Autodesk Inventor part; units mm, degrees
ref_plane "YZ Plane" through (0, 0, 0) normal (1, 0, 0) x (0, 1, 0)
ref_plane "XZ Plane" through (0, 0, 0) normal (0, 1, 0) x (-1, 0, 0)
ref_plane "XY Plane" through (0, 0, 0) normal (0, 0, 1) x (1, 0, 0)
sketch "Skizze1" plane through (0, 0, 0) normal (0, 0, 1) x (1, 0, 0)
  line L0 (-7, 0) -> (7, 0)
  line L1 (0, -7) -> (0, 7)
  circle A0 centre (0, 0) radius 5
  dimension "d0" = 10
extrude "Extrusion1" add sketch "Skizze1" along normal blind 82
sketch "Skizze2" plane through (0, 0, 82) normal (0, 0, 1) x (1, 0, 0)
  circle A0 centre (0, 0) radius 5
  circle A1 centre (0, 0) radius 2
  dimension "d3" = 4
extrude "Extrusion2" add sketch "Skizze2" along normal blind 6 contours A1
thread "Gewinde1"
sketch "Skizze3" plane through (0, 0, 0) normal (0, 0, -1) x (-1, 0, 0)
  circle A0 centre (0, 0) radius 5
  circle A1 centre (0, 0) radius 2
hole "Bohrung1" at (0, 0, 0) direction (0, 0, 1) diameter 4.134 depth 14.2 tip angle 118
properties part number "24_0497_0011"
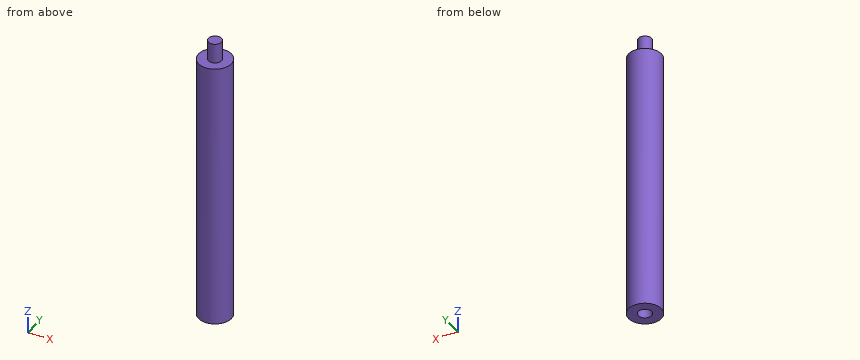
Here's how the part is built. I have some questions about the finished solid (model axes, mm). Coordinates: 2 decimals unless noted, no trailing zeros. Loops run counter-clockwise (first coordinate to the right, second up) from the corner with the lowest first, then second, coordinate; pieces in that order, holes last. Notation, with made-up numbers: (45.5, 22.25) -> (78.5, 22.25) arc R22 cw to (78.5, 29.25) -> close; hole circle Ø10 at (47, 70). An arc over 180 degrees is marked (long way). Return JSON: item names as keys, results as strings.
1) If we section it at A-A, the plane y = 3: Write out the boundary of the cut face in (x, z).
Results below:
{"outline": "(-4, 0) -> (4, 0) -> (4, 82) -> (-4, 82) -> close"}
2) If we section it at C-C, the plane z = 72.5: Write out the boundary of the cut face in (x, y), then the cut area to 3 significant figures.
Results below:
{"outline": "circle Ø10 at (0, 0)", "area": "78.5 mm²"}
3) Will these pins go through, and if not, where does the flat tip stop? pin 1 (4 mm diameter, centred on y = 3.5, z = 59.5, fed in from +X); pin 2 (5 mm diameter, centred on x = 3, z = 26.5, fed in from -Y); pin 3 (1 mm diameter, centred on y = -1, z = 13, fed in from +X).
Results below:
{"pin 1": "x = 4.77", "pin 2": "y = -4.97", "pin 3": "x = 4.97"}
4) I need wall thicknesses on line 1 (Z direction, x = 2.75, y = 3); line 2 (X direction, y = 1.75, z = 12). Which ranges of each line are inside material? Lowest first, please. Write a range as from..to.
Results below:
{"line 1": "0..82", "line 2": "-4.68..-1.1, 1.1..4.68"}
